Here's how the part is built. I have some questions about the finished solid (model axes, mm). Face numbers are marked on the shaded views. A direction names the side the tool comes from. Round coordinates to 2 decimals unless told otherwise and drop trailing zeros. Order: outer loops, then holes, each group sorted by start corner. A loop starts at its lowest first (then second) coordinate and runs counter-clockwise, first axis right, second up. Notation, with made-up numbers: (-0.75, -23) -> (18.25, -23) arc R7 cw to (18.25, -17) -> close; hole circle Ø4 at (66, 36.25). An arc over 180 degrees is marked (long way). Use a Markdown table: item, result. Add a question column.
(1) If I drill on probe 1 along Z at (x, y) = (7.25, 2.3); probe 2 along Y at (x, z) = (3, 3.35), over which ranges is the centre line in solid material (lowest first)?
(2) I want a section at C-C, the plane z = 4.05. Please give me the cut outline in (x, y).
(3) I want a section at B-B, the plane x = 4. Please give me the cut outline in (y, z), then the cut area to 3 significant figures.
(4) I'm going to push a flat-ended pin straight in: P1, Ø3.5, axis at x = 3.5, z = 2, coming from the -Y side. Where does the tip first touch, or does it pass through?
(5) On a 3-axis mill with a long thin cutter (end or side, diameter ignored), from which of +Z, -Z, +X, -X, +Y, -Y can I reach the whole of each face in a straight line? I mean the marked faces 1 and 2. Say none if no direction works.
(6) I want a section at A-A, the plane y = 2. Please give me the cut outline in (x, z), then the cut area to 3 significant figures.
(7) Thinking about a two-plate mould opening in Z: for the marked faces 3, 4 and 5, which applies, pulls with the +Z half, pulls with the -Z half, needs draft (parallel to the pull), parting line crosses it, or undercut?
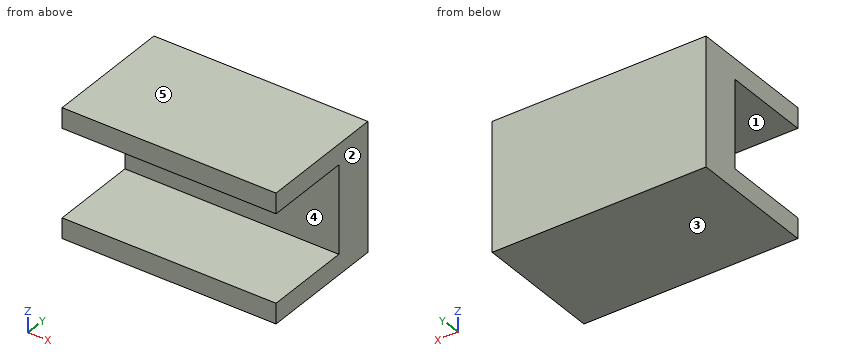
from build123d import *

# Parameters (mm, degrees)
F0_W     = 10
F0_H     = 6
F1_DEPTH = 6
F2_W     = 4.1
F2_H     = 4.1
F3_DEPTH = 10


with BuildPart() as f1:
    # F0 (on Top) → F1 (new body)
    with BuildSketch(Plane.XY):
        with Locations((5, 3)):
            Rectangle(F0_W, F0_H)
    extrude(amount=F1_DEPTH)

    # F2 (on face) → F3 (cut, through all)
    with BuildSketch(Plane.YZ.offset(10)):
        with Locations((2.05, 3)):
            Rectangle(F2_W, F2_H)
    extrude(amount=-F3_DEPTH, mode=Mode.SUBTRACT)


solid = f1.part
Taken from the geometry:
| question | item | result |
|---|---|---|
| 1 | probe 1 | z = 0 to 0.95, 5.05 to 6 |
| 1 | probe 2 | y = 4.1 to 6 |
| 2 | outline | (0, 4.1) -> (10, 4.1) -> (10, 6) -> (0, 6) -> close |
| 3 | outline | (0, 0) -> (6, 0) -> (6, 6) -> (0, 6) -> (0, 5.05) -> (4.1, 5.05) -> (4.1, 0.95) -> (0, 0.95) -> close |
| 3 | area | 19.2 mm2 |
| 4 | P1 | stops at y = 0 |
| 5 | face 1 | +X, -X, -Y |
| 5 | face 2 | +Z, -Z, +X, +Y, -Y |
| 6 | outline | (0, 0) -> (10, 0) -> (10, 0.95) -> (0, 0.95) -> close; (0, 5.05) -> (10, 5.05) -> (10, 6) -> (0, 6) -> close |
| 6 | area | 19.0 mm2 |
| 7 | face 3 | pulls with the -Z half |
| 7 | face 4 | undercut |
| 7 | face 5 | pulls with the +Z half |
